from build123d import *

# Parameters (mm, degrees)
SKETCH1_R            = 1.5
BOSS_EXTRUDE1_DEPTH  = 5
SKETCH2_R            = 2
BOSS_EXTRUDE13_DEPTH = 50
FILLET3_R            = 10
FILLET8_R            = 7.5
BOSS_EXTRUDE14_DEPTH = 5
FILLET9_R            = 7.5


with BuildPart() as part:
    # Sketch1 → Boss-Extrude1 (new body)
    with BuildSketch(Plane(origin=(0, 0, 0), x_dir=(1, 0, 0), z_dir=(0, 1, 0))):
        with BuildLine():
            Line((-7.071067812, -7.071067812), (-17.67766953, -17.67766953))
            Line((-17.67766953, -17.67766953), (-24.748737342, -10.606601718))
            Line((-24.748737342, -10.606601718), (-31.819805153, -17.67766953))
            Line((-31.819805153, -17.67766953), (-24.748737342, -24.748737342))
            ThreePointArc((-24.748737342, -24.748737342), (-17.67766953, -27.67766953), (-10.606601718, -24.748737342))
            Line((-10.606601718, -24.748737342), (-6.464466135, -20.606601758))
            ThreePointArc((-6.464466135, -20.606601758), (-3.220232647, -18.438874245), (0.606601677, -17.67766957))
            Line((0.606601677, -17.67766957), (154.3, -17.67766957))
            ThreePointArc((154.3, -17.67766957), (171.97766953, 0), (154.3, 17.67766953))
            Line((154.3, 17.67766953), (0.606601718, 17.67766953))
            ThreePointArc((0.606601718, 17.67766953), (-3.220232606, 18.438874205), (-6.464466094, 20.606601718))
            Line((-6.464466094, 20.606601718), (-10.606601718, 24.748737342))
            ThreePointArc((-10.606601718, 24.748737342), (-17.67766953, 27.67766953), (-24.748737342, 24.748737342))
            Line((-24.748737342, 24.748737342), (-31.819805153, 17.67766953))
            Line((-31.819805153, 17.67766953), (-24.748737342, 10.606601718))
            Line((-24.748737342, 10.606601718), (-17.67766953, 17.67766953))
            Line((-17.67766953, 17.67766953), (-7.071067812, 7.071067812))
            ThreePointArc((-7.071067812, 7.071067812), (-4.142135624, 0), (-7.071067812, -7.071067812))
        make_face()
        with Locations(Location((146.3, 0, 0), (0, 0, 270))):
            Circle(SKETCH1_R, mode=Mode.SUBTRACT)
        with Locations(Location((154.3, -8, 0), (0, 0, 270))):
            Circle(SKETCH1_R, mode=Mode.SUBTRACT)
        with Locations(Location((162.3, 0, 0), (0, 0, 270))):
            Circle(SKETCH1_R, mode=Mode.SUBTRACT)
        with Locations(Location((154.3, 8, 0), (0, 0, 270))):
            Circle(SKETCH1_R, mode=Mode.SUBTRACT)
        with BuildLine():
            Line((15.969736075, 11.850725041), (34.90716028, 1.868680325))
            ThreePointArc((34.90716028, 1.868680325), (35.606601718, 1.695624813), (36.306043156, 1.868680325))
            Line((36.306043156, 1.868680325), (55.24346736, 11.850725041))
            ThreePointArc((55.24346736, 11.850725041), (56.000119452, 13.537935589), (54.544025922, 14.67766953))
            Line((54.544025922, 14.67766953), (16.669177513, 14.67766953))
            ThreePointArc((16.669177513, 14.67766953), (15.213083984, 13.537935589), (15.969736075, 11.850725041))
        make_face(mode=Mode.SUBTRACT)
        with BuildLine():
            Line((50.969736075, 4.326944488), (69.90716028, 14.308989205))
            ThreePointArc((69.90716028, 14.308989205), (70.606601718, 14.482044716), (71.306043156, 14.308989205))
            Line((71.306043156, 14.308989205), (90.24346736, 4.326944488))
            ThreePointArc((90.24346736, 4.326944488), (91.000119452, 2.63973394), (89.544025922, 1.5))
            Line((89.544025922, 1.5), (51.669177513, 1.5))
            ThreePointArc((51.669177513, 1.5), (50.213083984, 2.63973394), (50.969736075, 4.326944488))
        make_face(mode=Mode.SUBTRACT)
        with BuildLine():
            Line((85.969736075, 11.850725041), (104.90716028, 1.868680325))
            ThreePointArc((104.90716028, 1.868680325), (105.606601718, 1.695624813), (106.306043156, 1.868680325))
            Line((106.306043156, 1.868680325), (125.24346736, 11.850725041))
            ThreePointArc((125.24346736, 11.850725041), (126.000119452, 13.537935589), (124.544025922, 14.67766953))
            Line((124.544025922, 14.67766953), (86.669177513, 14.67766953))
            ThreePointArc((86.669177513, 14.67766953), (85.213083984, 13.537935589), (85.969736075, 11.850725041))
        make_face(mode=Mode.SUBTRACT)
        with BuildLine():
            Line((120.969736075, 4.326944488), (138.40716028, 13.518329033))
            ThreePointArc((138.40716028, 13.518329033), (139.881468753, 13.475744727), (140.606601718, 12.191384545))
            Line((140.606601718, 12.191384545), (140.606601718, 3))
            ThreePointArc((140.606601718, 3), (140.16726189, 1.939339828), (139.106601718, 1.5))
            Line((139.106601718, 1.5), (121.669177513, 1.5))
            ThreePointArc((121.669177513, 1.5), (120.213083984, 2.63973394), (120.969736075, 4.326944488))
        make_face(mode=Mode.SUBTRACT)
        with BuildLine():
            Line((140.606601718, -12.191384545), (140.606601718, -3))
            ThreePointArc((140.606601718, -3), (140.16726189, -1.939339828), (139.106601718, -1.5))
            Line((139.106601718, -1.5), (121.669177513, -1.5))
            ThreePointArc((121.669177513, -1.5), (120.213083984, -2.63973394), (120.969736075, -4.326944488))
            Line((120.969736075, -4.326944488), (138.40716028, -13.518329033))
            ThreePointArc((138.40716028, -13.518329033), (139.881468753, -13.475744727), (140.606601718, -12.191384545))
        make_face(mode=Mode.SUBTRACT)
        with BuildLine():
            Line((124.544025922, -14.67766953), (86.669177513, -14.67766953))
            ThreePointArc((86.669177513, -14.67766953), (85.213083984, -13.537935589), (85.969736075, -11.850725041))
            Line((85.969736075, -11.850725041), (104.90716028, -1.868680325))
            ThreePointArc((104.90716028, -1.868680325), (105.606601718, -1.695624813), (106.306043156, -1.868680325))
            Line((106.306043156, -1.868680325), (125.24346736, -11.850725041))
            ThreePointArc((125.24346736, -11.850725041), (126.000119452, -13.537935589), (124.544025922, -14.67766953))
        make_face(mode=Mode.SUBTRACT)
        with BuildLine():
            Line((71.306043156, -14.308989205), (90.24346736, -4.326944488))
            ThreePointArc((90.24346736, -4.326944488), (91.000119452, -2.63973394), (89.544025922, -1.5))
            Line((89.544025922, -1.5), (51.669177513, -1.5))
            ThreePointArc((51.669177513, -1.5), (50.213083984, -2.63973394), (50.969736075, -4.326944488))
            Line((50.969736075, -4.326944488), (69.90716028, -14.308989205))
            ThreePointArc((69.90716028, -14.308989205), (70.606601718, -14.482044716), (71.306043156, -14.308989205))
        make_face(mode=Mode.SUBTRACT)
        with BuildLine():
            Line((36.306043156, -1.868680325), (55.24346736, -11.850725041))
            ThreePointArc((55.24346736, -11.850725041), (56.000119452, -13.537935589), (54.544025922, -14.67766953))
            Line((54.544025922, -14.67766953), (16.669177513, -14.67766953))
            ThreePointArc((16.669177513, -14.67766953), (15.213083984, -13.537935589), (15.969736075, -11.850725041))
            Line((15.969736075, -11.850725041), (34.90716028, -1.868680325))
            ThreePointArc((34.90716028, -1.868680325), (35.606601718, -1.695624813), (36.306043156, -1.868680325))
        make_face(mode=Mode.SUBTRACT)
    extrude(amount=BOSS_EXTRUDE1_DEPTH)

    # Sketch2 → Boss-Extrude13 (add)
    with BuildSketch(Plane.XZ):
        with BuildLine():
            Line((2.121320344, 0), (-18.384776311, 20.506096654))
            Line((-18.384776311, 20.506096654), (-26.516504294, 12.374368671))
            ThreePointArc((-26.516504294, 12.374368671), (-31.642135624, 0), (-26.516504294, -12.374368671))
            Line((-26.516504294, -12.374368671), (-18.384776311, -20.506096654))
            Line((-18.384776311, -20.506096654), (2.121320344, 0))
        make_face()
        Polygon((-24.748737342, -10.606601718), (-24.748737342, 10.606601718), (-21.213203436, 14.142135624), (-17.67766953, 17.67766953), (0, 0), (-17.67766953, -17.67766953), (-21.213203436, -14.142135624), align=None, mode=Mode.SUBTRACT)
        Polygon((-21.213203436, 14.142135624), (-24.748737342, 10.606601718), (-24.748737342, -10.606601718), (-21.213203436, -14.142135624), (-17.67766953, -17.67766953), (0, 0), (-17.67766953, 17.67766953), align=None)
        with Locations(Location((-17.67766953, -10.606601718, 0), (0, 0, 270))):
            Circle(SKETCH2_R, mode=Mode.SUBTRACT)
        with Locations(Location((-17.67766953, 10.606601718, 0), (0, 0, 270))):
            Circle(SKETCH2_R, mode=Mode.SUBTRACT)
    extrude(amount=BOSS_EXTRUDE13_DEPTH)

    # Fillet3
    fillet3_edges = [part.edges().sort_by_distance(p)[0] for p in [
        (2.121320344, -25, 0),
    ]]
    fillet(fillet3_edges, radius=FILLET3_R)

    # Fillet8
    fillet8_edges = [part.edges().sort_by_distance(p)[0] for p in [
        (-11.66726189, 0, 13.788582233),
        (-11.66726189, 0, -13.788582233),
        (-2.02081528, 0, 0),
    ]]
    fillet(fillet8_edges, radius=FILLET8_R)

    # Sketch3 → Boss-Extrude14 (add)
    with BuildSketch(Plane.XZ.offset(50)):
        with BuildLine():
            Line((-7.071067812, -7.071067812), (-17.67766953, -17.67766953))
            Line((-17.67766953, -17.67766953), (-24.748737342, -10.606601718))
            Line((-24.748737342, -10.606601718), (-31.819805153, -17.67766953))
            Line((-31.819805153, -17.67766953), (-24.760321052, -24.737153631))
            ThreePointArc((-24.760321052, -24.737153631), (-17.68925324, -27.666085819), (-10.618185428, -24.737153631))
            Line((-10.618185428, -24.737153631), (7.059484102, -7.059484102))
            ThreePointArc((7.059484102, -7.059484102), (9.98841629, 0.01158371), (7.059484102, 7.082651522))
            Line((7.059484102, 7.082651522), (-10.606601718, 24.748737342))
            ThreePointArc((-10.606601718, 24.748737342), (-17.67766953, 27.67766953), (-24.748737342, 24.748737342))
            Line((-24.748737342, 24.748737342), (-31.819805153, 17.67766953))
            Line((-31.819805153, 17.67766953), (-24.748737342, 10.606601718))
            Line((-24.748737342, 10.606601718), (-17.67766953, 17.67766953))
            Line((-17.67766953, 17.67766953), (-7.071067812, 7.071067812))
            ThreePointArc((-7.071067812, 7.071067812), (-4.142135624, 0), (-7.071067812, -7.071067812))
        make_face()
    extrude(amount=BOSS_EXTRUDE14_DEPTH)

    # Fillet9
    fillet9_edges = [part.edges().sort_by_distance(p)[0] for p in [
        (-11.66726189, -50, 13.788582233),
        (-11.66726189, -50, -13.788582233),
        (-2.02081528, -50, 0),
    ]]
    fillet(fillet9_edges, radius=FILLET9_R)


solid = part.part
CAD build for the part. Positions are in the model's coordinates, mm. A direction names the side the tool comes from. Give positions to 0.01 mm unless a question says otherwise; leave off trailing zeros. Write each loop counter-clockwise with the first axis right and the second up, starting at its lowest first coordinate (ties: lowest second). Pieces come first, ordered by that corner, then holes. Notation, with made-up numbers: (-16.75, 8.5) -> (-6.75, 8.5) arc R17 cw to (-6.75, 23.5) -> close; hole circle Ø8 at (27.5, 89). An arc over 180 degrees is marked (long way). Return JSON: item names as keys, results as strings.
Item 1: Band-saw the part on B-B (x = 94). List the corners of the cut face in (y, z).
Answer below:
{"outline": "(0, -17.68) -> (5, -17.68) -> (5, -14.68) -> (0, -14.68) -> close; (0, -7.62) -> (5, -7.62) -> (5, 7.62) -> (0, 7.62) -> close; (0, 14.68) -> (5, 14.68) -> (5, 17.68) -> (0, 17.68) -> close"}
Item 2: Two-plate mould, pull along X, no slides. Class faces 6 (the cylindrical face through (-2.02, -25.25, 0.11)), 7 (the cylindrical face through (-17.799, -52.465, -27.665)), 8 (the flat face through (25.306, 2.465, 6.93)): +X half, -X half, draft (parallel to the pull), parting line (faces both ways), or undercut.
Answer below:
{"face 6": "+X half", "face 7": "parting line", "face 8": "undercut"}
Item 3: Tool access for faces 1 (the flat face through (131, 2, -1.5)), 2 (the cylindrical face through (-4.143, -52.465, 0.11)), 3 (the flat face through (-28.2, 2.5, -21.3)), 4 (the cylindrical face through (-10.25, -2.26, 15.39)), 5 (the flat face through (-1.9, -52.46, -16.02)): list every direction of +Z, -Z, +X, -X, +Y, -Y with a clear straight run to the whole face (end or side of a thin tool).
Answer below:
{"face 1": "+Y, -Y", "face 2": "-X, -Y", "face 3": "-Z, -X, +Y, -Y", "face 4": "+Z, +X", "face 5": "-Z, +X, -Y"}
Item 4: Band-saw the part on A-A (y = -18). List the corners of the cut face in (x, z).
Answer below:
{"outline": "(-26.52, -12.37) -> (-18.38, -20.51) -> (-4.95, -7.07) arc R10 ccw to (-4.95, 7.07) -> (-18.38, 20.51) -> (-26.52, 12.37) arc R17.5 ccw to start; hole circle Ø4 at (-17.68, -10.61); hole circle Ø4 at (-17.68, 10.61)"}
Item 5: Drill centre lines: probe 1 along X at (y, z) = (2, 0); probe 2 along Z at (x, y) = (154.3, 3.95); probe 3 along Y at (x, z) = (-17, -23.5). Where is each one in solid material? Low to high.
Answer below:
{"probe 1": "x = -4.14 to 144.8, 147.8 to 160.8, 163.8 to 171.98", "probe 2": "z = -17.68 to -9.5, -6.5 to 6.5, 9.5 to 17.68", "probe 3": "y = -55 to -50, 0 to 5"}
Item 6: Band-saw the part on C-C (x = 46.5). List the corners of the cut face in (y, z).
Answer below:
{"outline": "(0, -17.68) -> (5, -17.68) -> (5, -14.68) -> (0, -14.68) -> close; (0, -7.24) -> (5, -7.24) -> (5, 7.24) -> (0, 7.24) -> close; (0, 14.68) -> (5, 14.68) -> (5, 17.68) -> (0, 17.68) -> close"}
Item 7: Drop flat-ended pins along their axis: pin 1 (2.5 mm diameter, centred on x = 107.5, y = 1.5, fed in from +Z); pin 2 (16.5 mm diameter, centred on x = 88.5, z = -11, fed in from -Y); pin 3 (5 mm diameter, centred on x = -17.68, z = -10.61, fed in from -Y); pin 4 (6 mm diameter, centred on x = 50.5, z = 21.5, fed in from +Y). Give the stop position or say it passes through.
Answer below:
{"pin 1": "stops at z = 17.68", "pin 2": "stops at y = 0", "pin 3": "stops at y = -50", "pin 4": "passes through"}
